Geometry check sheet. Reference: the model listing, model coordinates, mm. A direction names the side the tool comes from. Give positions to 0.01 mm unless a question says otherwise; leave off trailing zeros. Write each loop counter-clockwise with the first axis right and the second up, starting at its lowest first coordinate (ties: lowest second). Pieces come first, ordered by that corner, then holes. Notation, with made-up numbers: (64.25, -36) - (100.25, -36) arc R17 ccw to (100.25, -5) - close; hole circle Ø6 at (61, 2). An arc over 180 degrees is marked (long way). One line per question, with ' | ' between items. Start each with the question number.
Q1. Thickness scan on L1, parallel to Z at x = 10.25, y = 1.75; L2, parallel to Y at x = 11, z = 15.85; L3, parallel to Y at x = 1.75, z = 7.25. Record the ranges inside material, lowest first. Write a range as [from, to].
Q2. Section check A-A on x = 0. Record the boundary of the cut face in (y, z) (3 decimals).
Q3. Section check B-B on y = -10. Record the boundary of the cut face in (x, z).
Q4. Section check D-D on x = 11. Record the boundary of the cut face in (y, z).
Q5. Release check for a two-part mould opening along X. For faces 4 (the face through (-14.985, 0.66, 15.279)), 5 (the face through (1.3, -1.3, 6.8)), 6 (the face through (-4, 4, 13.8)) record: +X half, -X half, draft (parallel to the pull), parting line (faces both ways), or undercut.
Q6. Set-up check for faces 1 (the face through (-3, 0, 12)), 2 (the face through (3.908, 2.997, 6.803)), 3 (the face through (9.6, 0.06, 15.28)): record each of +Z, -Z, +X, -X, +Y, -Y from which the full face is reachable in a straight line by a thin tool's end or side.
Q7. Section check C-C on z = 5.25. Record the boundary of the cut face in (x, y) (3 decimals), and give its area (3 significant figures).
Q8. Gauge pin test, flat ends, axial feed: P1, Ø5, axis at x = 0, y = 0, coming from the +Z side; P2, Ø2, axis at y = -10, z = 13, coming from the -X side; P3, Ø8, axis at x = 0, y = 0, coming from the +Z side; P4, Ø1.5, axis at y = -2.5, z = 2, coming from the -X side. Record the tip position at first contact, or that the pin passes through.
```python
from build123d import *

# Parameters (mm, degrees)
SKETCH_1_R          = 4.925
SKETCH_1_R_2        = 1.55
EXTRUDE_1_DEPTH     = 13.8
SKETCH_2_R          = 15
SKETCH_2_R_2        = 1.4
SKETCH_2_R_3        = 1.15
SKETCH_2_R_4        = 1.55
EXTRUDE_2_DEPTH     = 3
SKETCH_3_R          = 3
CUT_EXTRUDE_1_DEPTH = 10


with BuildPart() as part:
    # 草图1 → 凸台-拉伸1 (new body)
    with BuildSketch(Plane.XY):
        with Locations(Location((0, 0, 0), (0, 0, 180))):
            Circle(SKETCH_1_R)
        with Locations(Location((0, 0, 0), (0, 0, 180))):
            Circle(SKETCH_1_R_2, mode=Mode.SUBTRACT)
    extrude(amount=EXTRUDE_1_DEPTH)

    # 草图2 → 凸台-拉伸2 (add)
    with BuildSketch(Plane.XY.offset(13.8)):
        Circle(SKETCH_2_R)
        with Locations((-11, 0)):
            Circle(SKETCH_2_R_2, mode=Mode.SUBTRACT)
        with Locations((0, 11)):
            Circle(SKETCH_2_R_2, mode=Mode.SUBTRACT)
        with Locations((11, 0)):
            Circle(SKETCH_2_R_2, mode=Mode.SUBTRACT)
        with Locations((0, -11)):
            Circle(SKETCH_2_R_2, mode=Mode.SUBTRACT)
        with Locations((-5.656854249, 5.656854249)):
            Circle(SKETCH_2_R_3, mode=Mode.SUBTRACT)
        with Locations((5.656854249, 5.656854249)):
            Circle(SKETCH_2_R_3, mode=Mode.SUBTRACT)
        with Locations((5.656854249, -5.656854249)):
            Circle(SKETCH_2_R_3, mode=Mode.SUBTRACT)
        with Locations((-5.656854249, -5.656854249)):
            Circle(SKETCH_2_R_3, mode=Mode.SUBTRACT)
        with Locations(Location((0, 0, 0), (0, 0, 180))):
            Circle(SKETCH_2_R_4, mode=Mode.SUBTRACT)
    extrude(amount=EXTRUDE_2_DEPTH)

    # 草图3 → 切除-拉伸1 (cut)
    with BuildSketch(Plane.XY.offset(16.8)):
        Circle(SKETCH_3_R)
    extrude(amount=-CUT_EXTRUDE_1_DEPTH, mode=Mode.SUBTRACT)


solid = part.part
```
Working result:
1) L1: z = [13.8, 16.8] | L2: y = [-10.2, -1.4], [1.4, 10.2] | L3: y = [-4.6, -2.44], [2.44, 4.6]
2) outline: (-15, 13.8) - (-12.4, 13.8) - (-12.4, 16.8) - (-15, 16.8) - close; (-9.6, 13.8) - (-4.925, 13.8) - (-4.925, 0) - (-1.55, 0) - (-1.55, 6.8) - (-3, 6.8) - (-3, 16.8) - (-9.6, 16.8) - close; (1.55, 0) - (4.925, 0) - (4.925, 13.8) - (9.6, 13.8) - (9.6, 16.8) - (3, 16.8) - (3, 6.8) - (1.55, 6.8) - close; (12.4, 13.8) - (15, 13.8) - (15, 16.8) - (12.4, 16.8) - close
3) outline: (-11.18, 13.8) - (-0.98, 13.8) - (-0.98, 16.8) - (-11.18, 16.8) - close; (0.98, 13.8) - (11.18, 13.8) - (11.18, 16.8) - (0.98, 16.8) - close
4) outline: (-10.2, 13.8) - (-1.4, 13.8) - (-1.4, 16.8) - (-10.2, 16.8) - close; (1.4, 13.8) - (10.2, 13.8) - (10.2, 16.8) - (1.4, 16.8) - close
5) face 4: parting line | face 5: undercut | face 6: draft
6) face 1: +Z | face 2: -Z | face 3: +Z, -Z
7) outline: circle Ø9.85 at (0, 0); hole circle Ø3.1 at (0, 0) | area: 68.7 mm2
8) P1: stops at z = 6.8 | P2: stops at x = -11.69 | P3: stops at z = 16.8 | P4: stops at x = -4.6
